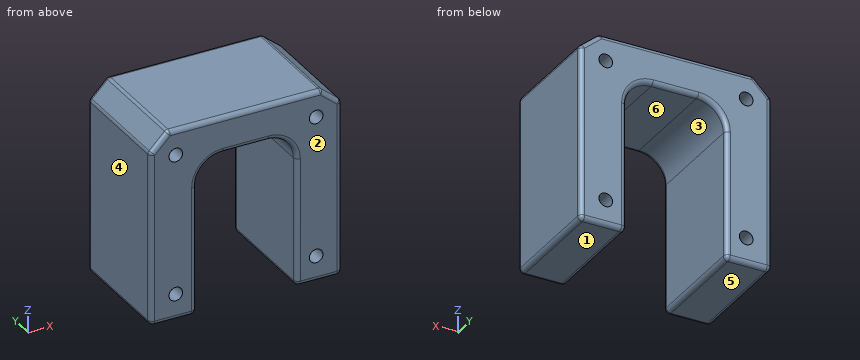
from build123d import *

# Parameters (mm, degrees)
BOSS_EXTRUDE1_DEPTH = 25
SKETCH2_R           = 1.5
CUT_EXTRUDE1_DEPTH  = 51.046074471
FILLET1_R           = 6
CUT_EXTRUDE2_DEPTH  = 51.046074471
FILLET2_R           = 1


with BuildPart() as part:
    # Sketch1 → Boss-Extrude1 (new body)
    with BuildSketch(Plane(origin=(0, 0, 0), x_dir=(1, 0, 0), z_dir=(0, 1, 0))):
        Polygon((-10.255294708, 3.008405172), (11.744705292, 3.008405172), (11.744705292, 37.308405172), (21.894705292, 37.308405172), (21.894705292, 2.897143722), (21.894705292, -4.991594828), (-20.405294708, -4.991594828), (-20.405294708, 3.008405172), (-20.405294708, 37.419666622), (-10.255294708, 37.419666622), align=None)
    extrude(amount=BOSS_EXTRUDE1_DEPTH)

    # Sketch2 → Cut-Extrude1 (cut, through all)
    with BuildSketch(Plane.XZ):
        with Locations(Location((-14.755294708, -31.658405172, 0), (0, 0, 270))):
            Circle(SKETCH2_R)
        with Locations(Location((-14.755294708, -0.658405172, 0), (0, 0, 270))):
            Circle(SKETCH2_R)
        with Locations(Location((16.244705292, -0.658405172, 0), (0, 0, 270))):
            Circle(SKETCH2_R)
        with Locations(Location((16.244705292, -31.658405172, 0), (0, 0, 270))):
            Circle(SKETCH2_R)
    extrude(amount=-CUT_EXTRUDE1_DEPTH, mode=Mode.SUBTRACT)

    # Fillet1
    fillet1_edges = [part.edges().sort_by_distance(p)[0] for p in [
        (-10.255294708, 12.5, -3.008405172),
        (11.744705292, 12.5, -3.008405172),
    ]]
    fillet(fillet1_edges, radius=FILLET1_R)

    # Sketch3 → Cut-Extrude2 (cut, through all)
    with BuildSketch(Plane.XZ):
        Polygon((21.894705292, 1.391259285), (17.527419638, 4.991594828), (21.894705292, 4.991594828), align=None)
        Polygon((-20.405294708, 0.994660971), (-16.397786785, 4.991594828), (-20.405294708, 4.991594828), align=None)
    extrude(amount=-CUT_EXTRUDE2_DEPTH, mode=Mode.SUBTRACT)

    # Fillet2
    fillet2_edges = [part.edges().sort_by_distance(p)[0] for p in [
        (16.819705292, 25, -37.308405172),
        (-15.330294708, 0, -37.419666622),
        (11.744705292, 0, -23.158405172),
        (16.819705292, 0, -37.308405172),
        (11.744705292, 25, -23.158405172),
        (-20.405294708, 12.5, -37.419666622),
        (-10.255294708, 12.5, -37.419666622),
        (11.744705292, 12.5, -37.308405172),
        (21.894705292, 12.5, -37.308405172),
        (-15.330294708, 25, -37.419666622),
        (-20.405294708, 25, -18.212502825),
        (-10.255294708, 0, -23.214035897),
        (-10.255294708, 25, -23.214035897),
        (0.744705292, 0, -3.008405172),
        (0.744705292, 25, -3.008405172),
        (-8.497935395, 0, -4.765764485),
        (-8.497935395, 25, -4.765764485),
        (9.98734598, 0, -4.765764485),
        (9.98734598, 25, -4.765764485),
        (21.894705292, 0, -17.958572944),
        (21.894705292, 25, -17.958572944),
        (19.711062465, 25, 3.191427056),
        (21.894705292, 12.5, 1.391259285),
        (17.527419638, 12.5, 4.991594828),
        (19.711062465, 0, 3.191427056),
        (0.564816427, 0, 4.991594828),
        (0.564816427, 25, 4.991594828),
        (-20.405294708, 12.5, 0.994660971),
        (-18.401540746, 25, 2.993127899),
        (-16.397786785, 12.5, 4.991594828),
        (-18.401540746, 0, 2.993127899),
        (-20.405294708, 0, -18.212502825),
    ]]
    fillet(fillet2_edges, radius=FILLET2_R)


solid = part.part
The listing builds one solid part. Answer for the finished solid, in the listing's coordinates (mm). Face numbers are marked on the shaded views. A direction names the side the tool comes from. Coordinates: 2 decimals unless noted, no trailing zeros. Order: outer loops, then holes, each group sorted by start corner. A loop starts at its lowest first (then second) coordinate and runs counter-clockwise, first axis right, second up. Notation, with made-up numbers: (-20.75, 68.25) -> (26.25, 68.25) arc R19 ccw to (26.25, 75.25) -> close; hole circle Ø2 at (71, 87). An arc over 180 degrees is marked (long way). Answer in a Markdown table with one row per item. Add a question column.
Item 1: Find section A-A (z = -23.5). Write down the section's boundary in (x, y).
Item 2: Each of these flat-tipped pins is pushed along its axis until it touches: P1, Ø4, axis at x = 18, y = 8.5, coming from the -Z side; P2, Ø1.8, axis at x = 16.24, z = -0.66, coming from the -Y side; P3, Ø8, axis at x = 0, y = 11.5, coming from the -Z side; P4, Ø3, axis at x = -5, y = 18.5, coming from the -Z side. Where does it stop, or does it pass through?
Item 3: Find section D-D (y = 13.5). Write down the section's boundary in (x, z), then the cut area to 3 significant figures.
Item 4: Find the intervals of material crossed by L1, parallel to X at y = 23.25, z = -31.5; L2, parallel to X at y = 10, z = -20; L3, parallel to X at y = 2, z = -30.5, in increasing order. Write a range as from..to.
Item 5: Find section B-B (z = -31). Write down the section's boundary in (x, y), then the cut area to 3 significant figures.
Item 6: Which of the six approach directions +Z, -Z, +X, -X, +Y, -Y give full straight-line access (tool end or side, diameter ignored) to the marked faces 1, 2 and 3?
Item 7: Find section C-C (x = -3). Write down the section's boundary in (y, z).
Item 8: Determine the mould class of the marked faces 4, 5 and 6 for opening direction X: +X half, -X half, draft (parallel to the pull), parting line (faces both ways), or undercut.
Result set:
| question | item | result |
|---|---|---|
| 1 | outline | (-20.41, 1) arc R1 ccw to (-19.41, 0) -> (-11.26, 0) arc R1 ccw to (-10.26, 1) -> (-10.26, 24) arc R1 ccw to (-11.26, 25) -> (-19.41, 25) arc R1 ccw to (-20.41, 24) -> close; (11.74, 1) arc R1 ccw to (12.74, 0) -> (20.89, 0) arc R1 ccw to (21.89, 1) -> (21.89, 24) arc R1 ccw to (20.89, 25) -> (12.74, 25) arc R1 ccw to (11.74, 24) -> close |
| 2 | P1 | stops at z = -37.31 |
| 2 | P2 | passes through |
| 2 | P3 | stops at z = -3.01 |
| 2 | P4 | stops at z = -3.44 |
| 3 | outline | (-20.41, -36.42) arc R1 ccw to (-19.41, -37.42) -> (-11.26, -37.42) arc R1 ccw to (-10.26, -36.42) -> (-10.26, -9.01) arc R6 cw to (-4.26, -3.01) -> (5.74, -3.01) arc R6 cw to (11.74, -9.01) -> (11.74, -36.31) arc R1 ccw to (12.74, -37.31) -> (20.89, -37.31) arc R1 ccw to (21.89, -36.31) -> (21.89, 0.92) arc R1 ccw to (21.53, 1.69) -> (17.8, 4.76) arc R1 ccw to (17.17, 4.99) -> (-15.98, 4.99) arc R1 ccw to (-16.69, 4.7) -> (-20.11, 1.29) arc R1 ccw to (-20.41, 0.58) -> close; hole circle Ø3 at (-14.76, -31.66); hole circle Ø3 at (-14.76, -0.66); hole circle Ø3 at (16.24, -31.66); hole circle Ø3 at (16.24, -0.66) |
| 3 | area | 1,010 mm² |
| 4 | L1 | x = -20.41..-16.25, -13.26..-10.26, 11.74..14.75, 17.74..21.89 |
| 4 | L2 | x = -20.41..-10.26, 11.74..21.89 |
| 4 | L3 | x = -20.41..-15.71, -13.8..-10.26, 11.74..15.29, 17.2..21.89 |
| 5 | outline | (-20.41, 1) arc R1 ccw to (-19.41, 0) -> (-16.1, 0) -> (-16.1, 25) -> (-19.41, 25) arc R1 ccw to (-20.41, 24) -> close; (-13.41, 0) -> (-11.26, 0) arc R1 ccw to (-10.26, 1) -> (-10.26, 24) arc R1 ccw to (-11.26, 25) -> (-13.41, 25) -> close; (11.74, 1) arc R1 ccw to (12.74, 0) -> (14.9, 0) -> (14.9, 25) -> (12.74, 25) arc R1 ccw to (11.74, 24) -> close; (17.59, 0) -> (20.89, 0) arc R1 ccw to (21.89, 1) -> (21.89, 24) arc R1 ccw to (20.89, 25) -> (17.59, 25) -> close |
| 5 | area | 371 mm² |
| 6 | face 1 | -Z, +X, +Y, -Y |
| 6 | face 2 | +Z, -Z, +X, -X, -Y |
| 6 | face 3 | -Z, +Y, -Y |
| 7 | outline | (0, -2.01) arc R1 ccw to (1, -3.01) -> (24, -3.01) arc R1 ccw to (25, -2.01) -> (25, 3.99) arc R1 ccw to (24, 4.99) -> (1, 4.99) arc R1 ccw to (0, 3.99) -> close |
| 8 | face 4 | -X half |
| 8 | face 5 | draft |
| 8 | face 6 | undercut |
